```python
from build123d import *

# Parameters (mm, degrees)
SKETCH1_W                = 70
SKETCH1_H                = 70
BOSS_EXTRUDE1_DEPTH      = 5
SKETCH2_W                = 5
SKETCH2_H                = 3
BOSS_EXTRUDE2_DEPTH      = 5
BOSS_EXTRUDE6_DEPTH      = 5
BOSS_EXTRUDE6_DEPTH_BACK = 5
SKETCH16_R               = 2
BOSS_EXTRUDE10_DEPTH     = 2


with BuildPart() as part:
    # Sketch1 → Boss-Extrude1 (new body)
    with BuildSketch(Plane(origin=(0, 0, 0), x_dir=(0, 1, 0), z_dir=(0, 0, 1))):
        Rectangle(SKETCH1_W, SKETCH1_H)
    extrude(amount=BOSS_EXTRUDE1_DEPTH)

    # Sketch2 → Boss-Extrude2 (add)
    with BuildSketch(Plane(origin=(0, 35, 0), x_dir=(-1, 0, 0), z_dir=(0, 1, 0))):
        with Locations((-15, 1.5)):
            Rectangle(SKETCH2_W, SKETCH2_H)
        with Locations((15, 1.5)):
            Rectangle(SKETCH2_W, SKETCH2_H)
    extrude(amount=BOSS_EXTRUDE2_DEPTH)

    # Sketch10 → Boss-Extrude6 (add, two sides: drawn at the far end of the back side and taken through both)
    with BuildSketch(Plane.YZ.offset(-BOSS_EXTRUDE6_DEPTH_BACK)):
        Polygon((20, 5), (-25, 45), (-35, 45), (-35, 5), align=None)
    extrude(amount=BOSS_EXTRUDE6_DEPTH + BOSS_EXTRUDE6_DEPTH_BACK)

    # Sketch16 → Boss-Extrude10 (add)
    with BuildSketch(Plane(origin=(0, 11.310344828, 12.724137931), x_dir=(1, 0, 0), z_dir=(0, 0.6643638388299197, 0.7474093186836598))):
        with Locations(Location((0, 1.62636718, 0), (0, 0, 270))):
            Circle(SKETCH16_R)
        with Locations(Location((0, -38.581605714, 0), (0, 0, 270))):
            Circle(SKETCH16_R)
    extrude(amount=BOSS_EXTRUDE10_DEPTH)


solid = part.part
```
CAD build for the part. Positions are in the model's coordinates, mm. A direction names the side the tool comes from. Coordinates: 2 decimals unless noted, no trailing zeros. Order: outer loops, then holes, each group sorted by start corner. A loop starts at its lowest first (then second) coordinate and runs counter-clockwise, first axis right, second up.
(1) Mould opens along Z. For faces 4 (the face through (0, 13.9, 13.1)), 5 (the face through (0, 2, 0)), 6 (the face through (-17.5, 37, 1)), 7 (the face through (0.601, 11.755, 13.648)) say: released by +Z, released by -Z, zero draft, split by the parting line, or undercut.
Solution:
face 4: released by +Z
face 5: released by -Z
face 6: zero draft
face 7: undercut
(2) Saw through at B-B, the plane z = 4. Write the cut outline in (x, y).
Solution:
outline: (-35, -35) - (35, -35) - (35, 35) - (-35, 35) - close
(3) Drill centre lines: L1, parallel to Z at x = 25, y = 12; L2, parallel to Y at x = -6, z = 2; L3, parallel to X at y = -25, z = 5.5. Where is each one in solid material? Low to high.
Solution:
L1: z = 0 to 5
L2: y = -35 to 35
L3: x = -5 to 5
(4) Pin check, flat tips, straight feed: pin 1 Ø4 at (x, y) = (14, 36.5) entering from +Z; pin 2 Ø0.9 at (y, z) = (38.5, 1) entering from +X; pin 3 Ø20 at (y, z) = (1.5, 32.5) entering from +X. Stop position of each tip, or through.
Solution:
pin 1: stops at z = 5
pin 2: stops at x = 17.5
pin 3: stops at x = 5
(5) Which spindle directions (+Z, -Z, +X, -X, +Y, -Y) get a long thin tool onto all of the face, cutting with end or side? Do faces 1 (the face through (-5, -14, 21)), 2 (the face through (15, 37, 3)), 3 (the face through (-12.5, 37, 1)). Say none if no direction does.
Solution:
face 1: +Z, -X, +Y, -Y
face 2: +Z, +X, -X, +Y
face 3: +Z, -Z, +Y
(6) Saw through at D-D, the plane y = 17. Write the cut outline in (x, z).
Solution:
outline: (-35, 0) - (35, 0) - (35, 5) - (5, 5) - (5, 7.67) - (-5, 7.67) - (-5, 5) - (-35, 5) - close
(7) Saw through at C-C, the plane x = -19.5. Write the cut outline in (y, z), and give its area (3 significant figures).
Solution:
outline: (-35, 0) - (35, 0) - (35, 5) - (-35, 5) - close
area: 350 mm2
(8) Saw through at A-A, the plane y = -1. Write the cut outline in (x, z), and give its area (3 significant figures).
Solution:
outline: (-35, 0) - (35, 0) - (35, 5) - (5, 5) - (5, 23.67) - (-5, 23.67) - (-5, 5) - (-35, 5) - close
area: 537 mm2
